from build123d import *
from build123d.topology import SkipClean

# Parameters (mm, degrees)
SKETCH1_R               = 101.6
BOSS_EXTRUDE1_DEPTH     = 25.4
SKETCH4_R               = 88.9
SKETCH4_R_2             = 83.82
BOSS_EXTRUDE2_DEPTH     = 50.8
CUT_EXTRUDE4_DEPTH      = 101.6
CUT_EXTRUDE4_DEPTH_BACK = 101.6
SKETCH2_R               = 9.525
FILLET7_R               = 12.7
FILLET8_R               = 3.81
SKETCH11_R              = 50.4825
SKETCH11_R_2            = 45.72
BOSS_EXTRUDE5_DEPTH     = 50.8
SKETCH13_W              = 8.068772826
SKETCH13_H              = 9.525
SKETCH14_R              = 5.08
CUT_EXTRUDE5_DEPTH      = 50.8


# Some blends are built 0.0001 mm under size
with BuildPart() as part:
    # Sketch1 → Boss-Extrude1 (new body)
    with BuildSketch(Plane(origin=(0, 0, 0), x_dir=(1, 0, 0), z_dir=(0, 1, 0))):
        with Locations(Location((0, 0, 0), (0, 0, 270))):
            Circle(SKETCH1_R)
    extrude(amount=BOSS_EXTRUDE1_DEPTH)

    # Sketch4 → Boss-Extrude2 (add)
    with BuildSketch(Plane(origin=(0, 25.4, 0), x_dir=(1, 0, 0), z_dir=(0, 1, 0))):
        with Locations(Location((0, 0, 0), (0, 0, 270))):
            Circle(SKETCH4_R)
        with Locations(Location((0, 0, 0), (0, 0, 270))):
            Circle(SKETCH4_R_2, mode=Mode.SUBTRACT)
    extrude(amount=BOSS_EXTRUDE2_DEPTH)

    # Sketch2 → Cut-Extrude4 (cut, two sides: drawn at the far end of the back side and taken through both)
    with BuildSketch(Plane(origin=(0, 0, 0), x_dir=(0, 0, -1), z_dir=(1, 0, 0)).offset(-CUT_EXTRUDE4_DEPTH_BACK)):
        with Locations(Location((50.8, 12.7, 0), (0, 0, 180))):
            Circle(SKETCH2_R)
        with Locations(Location((-50.8, 12.7, 0), (0, 0, 180))):
            Circle(SKETCH2_R)
    extrude(amount=CUT_EXTRUDE4_DEPTH + CUT_EXTRUDE4_DEPTH_BACK, mode=Mode.SUBTRACT)

    # Fillet7
    fillet7_edges = [part.edges().sort_by_distance(p)[0] for p in [
        (0, 25.4, -88.9),
    ]]
    fillet(fillet7_edges, radius=FILLET7_R - 0.0001)  # a hair under: the kernel refuses the full size

    # Fillet8
    # the kernel refuses this fillet: 3.81 mm, written as the material it takes off along each edge
    with BuildSketch(Plane(origin=(0, 25.4, 0), x_dir=(0, 0, 1), z_dir=(-1, 0, 0))) as fillet8_piece_1:
        with BuildLine():
            CenterArc((97.79, -3.364391457), FILLET8_R, 360, 76.657910561)
            Line((101.6, -3.364391457), (101.981, -3.364391457))
            Line((101.981, -3.364391457), (101.981, 0))
            Line((101.981, 0), (101.6, 0.381))
            ThreePointArc((101.6, 0.381), (101.5999, 0.381), (98.757134319, 0.713491843))
            Line((98.757134319, 0.713491843), (98.669213018, 0.34277518))
        make_face()
    revolve(axis=Axis((0, 25.4, 0), (0, 1, 0)), mode=Mode.SUBTRACT)

    # Sketch11 → Boss-Extrude5 (add)
    with SkipClean():  # the faces are left unmerged after this step: merging them gives an invalid solid
        with BuildSketch(Plane(origin=(0, 25.4, 0), x_dir=(1, 0, 0), z_dir=(0, 1, 0))):
            with Locations(Location((0, 0, 0), (0, 0, 270))):
                Circle(SKETCH11_R)
            with Locations(Location((0, 0, 0), (0, 0, 270))):
                Circle(SKETCH11_R_2, mode=Mode.SUBTRACT)
        extrude(amount=BOSS_EXTRUDE5_DEPTH)

    # Sketch13 → Revolve1 (revolve)
    with SkipClean():  # the faces are left unmerged after this step: merging them gives an invalid solid
        with BuildSketch(Plane.XY, mode=Mode.PRIVATE) as revolve1_sk:
            with Locations((41.685613587, 68.2625)):
                Rectangle(SKETCH13_W, SKETCH13_H)
        revolve(revolve1_sk.sketch.rotate(Axis((0, 80.01, 0), (0, -1, 0)), 90), axis=Axis((0, 80.01, 0), (0, -1, 0)))

    # Sketch14 → Cut-Extrude5 (cut)
    with SkipClean():  # the faces are left unmerged after this step: merging them gives an invalid solid
        with BuildSketch(Plane.XY):
            with Locations(Location((0, 50.8, 0), (0, 0, 90))):
                Circle(SKETCH14_R)
        extrude(amount=-CUT_EXTRUDE5_DEPTH, mode=Mode.SUBTRACT)


solid = part.part
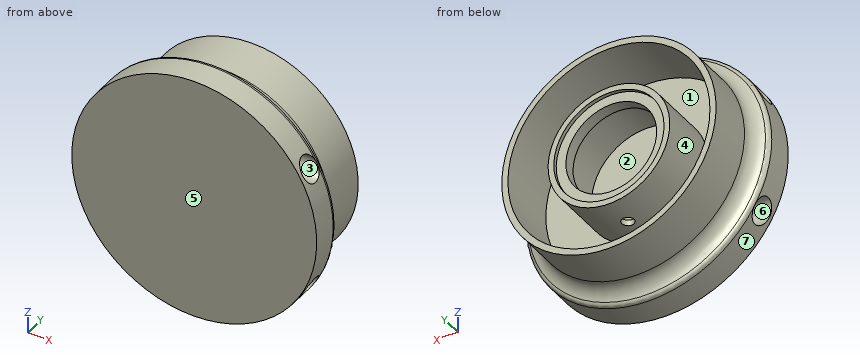
Verification items for the finished model (mm, model axes). Face numbers are marked on the shaded views. A direction names the side the tool comes from. Round coordinates to 2 decimals unless told otherwise and drop trailing zeros. Write each loop counter-clockwise with the first axis right and the second up, starting at its lowest first coordinate (ties: lowest second). Pieces come first, ordered by that corner, then holes.
(1) Section check B-B (x = 0). Give the number of separate pieces and of enclosed holes in the cut face, plus the area to 3 significant figures.
Returned:
separate pieces: 2
enclosed holes: 2
area: 5,760 mm2
(2) Mould release check, pull along Z, two halves, no side actions. Record for the marked faces 4, 5, 6 and 7: pulls with the +Z half, pulls with the -Z half, needs draft (parallel to the pull), parting line crosses it, or undercut.
Returned:
face 4: undercut
face 5: needs draft
face 6: undercut
face 7: parting line crosses it
(3) Material ranges on line 1 (X direction, y = 45.5, z = 0); line 2 (X direction, y = 70, z = 0); line 3 (Z direction, x = -29.5, y = 71), recorded low to high.
Returned:
line 1: x = -88.9 to -83.82, -50.48 to -45.72, 45.72 to 50.48, 83.82 to 88.9
line 2: x = -88.9 to -83.82, -50.48 to -37.65, 37.65 to 50.48, 83.82 to 88.9
line 3: z = -83.86 to -78.46, -40.97 to -23.4, 23.4 to 40.97, 78.46 to 83.86
(4) Access from +Z, -Z, +X, -X, +Y, -Y to the whole of each face (thin tool, end or side, straight path). Record for the marked faces 1, 2 and 3.
Returned:
face 1: +Y
face 2: none
face 3: +X, -X
(5) Depth check by flat-ended pin: pin 1 Ø6 at (x, y) = (0, 50.8) entering from -Z; pin 2 Ø1 at (y, z) = (60.5, 77.5) entering from +X; pin 3 Ø12 at (y, z) = (63, 46) entering from -X; pin 4 Ø3 at (x, z) = (-34.5, 75.5) entering from -Y. Enter the tip coordinate at first touch or a pass-through.
Returned:
pin 1: stops at z = -88.9
pin 2: stops at x = 44.43
pin 3: stops at x = -79.39
pin 4: stops at y = 0
(6) Section check A-A (y = 70). Enter the section's corners in (x, z) (1 decimal).
Returned:
outline: circle Ø177.8 at (0, 0); circle Ø101 at (0, 0); hole circle Ø167.6 at (0, 0); hole circle Ø75.3 at (0, 0)
(7) Section check D-D (y = 50.8). Enter the section's corners in (x, z) (1 decimal), plus the area to 3 significant figures.
Returned:
outline: circle Ø177.8 at (0, 0); (-5.1, -50.2) - (-5.1, -45.4) arc R45.7 cw (long way) to (5.1, -45.4) - (5.1, -50.2) arc R50.5 ccw (long way) to start; hole circle Ø167.6 at (0, 0)
area: 4,150 mm2
